Geometry: final body of the model. Coordinates: model frame, mm. A direction names the side the tool comes from. Round coordinates to 2 decimals unless told otherwise and drop trailing zeros. Loops run counter-clockwise (first coordinate to the right, second up) from the corner with the lowest first, then second, coordinate; pieces in that order, holes last. Notation, with made-up numbers: M 7.25,-23.75 L 11.25,-23.75 A25 cw 11.25,-6.75 Z; hole C 82,-12 d10. An arc over 180 degrees is marked long. Answer as a JSON object with one key per item and string values.
Autodesk Inventor part; units mm, degrees
ref_plane "YZ Plane" through (0, 0, 0) normal (1, 0, 0) x (0, 1, 0)
ref_plane "XZ Plane" through (0, 0, 0) normal (0, 1, 0) x (-1, 0, 0)
ref_plane "XY Plane" through (0, 0, 0) normal (0, 0, 1) x (1, 0, 0)
sketch "Sketch1" plane through (0, 0, 0) normal (1, 0, 0) x (0, 1, 0)
  circle A0 centre (0, 0) radius 14
  line L0 (-6.3479, 7.25) -> (-17.5, 7.25)
  line L1 (-17.5, 7.25) -> (-17.5, -7.25)
  line L2 (-17.5, -7.25) -> (-6.3479, -7.25)
  circle A1 centre (-0.0001, 17.5) radius 3.5
  circle A2 centre (-0.0001, 17.5) radius 2.1
  line L3 (3.4999, 17.5) -> (3.4999, 13.5555)
  line L4 (-3.5001, 17.5) -> (-3.4999, 13.5555)
  line L5 (-14, 0) -> (14, 0)
  circle A3 centre (-0.0001, -17.5) radius 3.5
  circle A4 centre (-0.0001, -17.5) radius 2.1
  line L6 (3.4999, -17.5) -> (3.4999, -13.5555)
  line L7 (-3.5001, -17.5) -> (-3.4999, -13.5555)
  point P0 (-11.9765, -7.25)
  point P1 (-11.9765, 7.25)
  dimension "d0" = 28
  dimension "d7" = 14.5
  dimension "d8" = 7.25
  dimension "d9" = 17.5
  dimension "d12" = 7
  dimension "d13" = 4.2
  dimension "d14" = 17.5
extrude "Extrusion1" add sketch "Sketch1" along normal blind 19 contours L5 A0 | A0 L5 | A0 L2 L1 L0
extrude "Extrusion2" add sketch "Sketch1" along normal blind 1 contours A0 A1 L3 | L6 A3 A0 | A0 L4 A1 | A1 | A3 L7 A0 | A3
sketch "Sketch3" plane through (19, 0, 0) normal (1, 0, 0) x (0, 0, -1)
  line L0 (0, 0) -> (0, 8)
  circle A0 centre (0, 8) radius 4.5
  circle A1 centre (0, 8) radius 2.5
  dimension "d17" = 8
  dimension "d18" = 9
  dimension "d19" = 5
extrude "Extrusion3" add sketch "Sketch3" along normal blind 1.5
extrude "Extrusion4" add sketch "Sketch3" along normal blind 2.5 contours A1
sketch "Sketch5" plane through (21.5, 8, 0) normal (1, 0, 0) x (0, 0, -1)
  circle A0 centre (0, 0) radius 2.5
  line L0 (-2, 1.5) -> (2, 1.5)
  circle A1 centre (0, 0) radius 2.5
  line L1 (-2.5, 0) -> (2.5, 0)
  line L2 (-2, -1.5) -> (2, -1.5)
  point P0 (0, -8)
  dimension "d24" = 1.5
extrude "Extrusion5" add sketch "Sketch5" along normal blind 6 contours L1 A0 L0 | A0 L2 L1
properties part number "motor"
1) Pin query (flat end, axial travel): P1, Ø5.5, axis at y = 0, z = -17.5, coming from the +X side; P2, Ø1.1, axis at x = 0.5, z = -16, coming from the -Y side; P3, Ø2, axis at x = 21.5, y = -8, coming from the -Z side; P4, Ø1, axis at x = 15.5, y = 9, coming from the -Z side. Return the tip coordinate at first contact, or that it passes through.
Results:
{"P1": "x = 1", "P2": "y = -3.5", "P3": "through", "P4": "z = -11.12"}
2) Section query C-C (y = 11.5). Return the cut outline in (x, z).
Results:
{"outline": "M 0,-7.98 L 19,-7.98 L 19,-2.83 L 20.5,-2.83 L 20.5,2.83 L 19,2.83 L 19,7.98 L 0,7.98 Z"}
3) Section query D-D (x = 4.5). Return the cut outline in (y, z).
Results:
{"outline": "M -17.5,-7.25 L -11.98,-7.25 A14 ccw long -11.98,7.25 L -17.5,7.25 Z"}
4) Section query B-B (z = 0). Return the cut outline in (x, y), and give its area (3 significant figures).
Results:
{"outline": "M 0,-17.5 L 19,-17.5 L 19,3.5 L 20.5,3.5 L 20.5,5.5 L 21.5,5.5 L 21.5,6.5 L 27.5,6.5 L 27.5,9.5 L 21.5,9.5 L 21.5,10.5 L 20.5,10.5 L 20.5,12.5 L 19,12.5 L 19,14 L 0,14 Z", "area": "635 mm2"}
5) Section query A-A (y = 0). Return the cut outline in (x, z), and give its area (3 significant figures).
Results:
{"outline": "M 0,-21 L 1,-21 L 1,-19.6 L 0,-19.6 Z; M 0,-15.4 L 1,-15.4 L 1,-14 L 19,-14 L 19,14 L 1,14 L 1,15.4 L 0,15.4 Z; M 0,19.6 L 1,19.6 L 1,21 L 0,21 Z", "area": "538 mm2"}
6) Reachability of faces 1 (the flat face through (9, -15, 7.25)), 2 (the flat face through (21.5, 6, 0)), 3 (the flat face through (24, 9.5, 0)), 4 (the flat face through (9, -15, -7.25)), 5 (the cylindrical face through (9.37, 13.99, 0.51)) from +Z, -Z, +X, -X, +Y, -Y: full face, straight path, thin tool, end or side. Return the list, or none.
Results:
{"face 1": "+Z, +X, -X, -Y", "face 2": "+Z, -Z, +X, -Y", "face 3": "+Z, -Z, +X, +Y", "face 4": "-Z, +X, -X, -Y", "face 5": "+X"}
7) Pull-direction query (Y, two-part tool) for faces 6 (the cylindrical face through (0.493, -0.273, 15.418)), 7 (the flat face through (20.5, 6, -2)), 8 (the flat face through (9, -17.5, 0)); classes: +Y half, -Y half, draft (parallel to the pull), parting line (faces both ways), or undercut.
Results:
{"face 6": "undercut", "face 7": "draft", "face 8": "-Y half"}
8) Ray query, line 1 (X direction, y = -2, z = -10.5); line 2 (Z direction, x = 8.5, y = -12); line 3 (X direction, y = 9, z = 3). Return the intervals inside material, ascending.
Results:
{"line 1": "0 to 19", "line 2": "-7.25 to 7.25", "line 3": "0 to 20.5"}
